Model file for the job. Use its own axes, mm. A direction names the side the tool comes from. Give positions to 0.01 mm unless a question says otherwise; leave off trailing zeros. Order: outer loops, then holes, each group sorted by start corner. A loop starts at its lowest first (then second) coordinate and runs counter-clockwise, first axis right, second up. Notation, with made-up numbers: M -40,43.25 L -2,43.25 A18 cw -2,69.25 Z; hole C -31,36.5 d4. An arc over 180 degrees is marked long. Return JSON: item names as keys, results as strings. Group by question number.
1. 3-axis set-ups, long thin cutter, end or side, ignore diameter. For faces 1 (the face through (0.33, 96.48, -19.07)), 2 (the face through (0, 41, -14)), 3 (the face through (-10, 63, -11)): which of +Z, -Z, +X, -X, +Y, -Y reach the whole face in a straight line?
2. Slice it at C-C on y = 77.5. List the corners of the cut face in (x, z).
3. Wall check: probe 1 along Y at (x, z) = (0, -3.25); probe 2 along Y at (x, z) = (0, -19.25); probe 3 along X at (y, z) = (21, -12). Give the ranges that are in metal, low to high. Write a range as [from, to].
4. Slice it at D-D on x = -4. List the corners of the cut face in (y, z).
5. Slice it at A-A on x = 0. List the corners of the cut face in (y, z).
6. Slice it at B-B on z = -17. List the corners of the cut face in (x, y), then the cut area to 3 significant figures.
7. Pin check, flat tips, straight feed: pin 1 (8 mm diameter, centred on y = 35.5, z = -10.5, fed in from +X); pin 2 (6 mm diameter, centred on x = -4.5, y = 33.5, fed in from -Z); pin 3 (3 mm diameter, centred on y = 57, z = -16.5, fed in from -X); pin 4 (4 mm diameter, centred on x = -13.5, y = 31, fed in from -Z). Stop position of each tip, or through.
8. Two-plate mould, pull along Y, no slides. Class faces 4 (the face through (0, 94, -14)), 5 (the face through (0, 0, -7)), 6 (the face through (13, 51, -6)): released by +Y, released by -Y, zero draft, split by the parting line, or undercut.
from build123d import *

# Parameters (mm, degrees)
DODANIE_WYCI_GNI_CIE1_DEPTH = 104
SZKIC2_W                    = 20
SZKIC2_H                    = 20
DODANIE_WYCI_GNI_CIE2_DEPTH = 10
SZKIC3_R                    = 2.5
WYTNIJ_WYCI_GNI_CIE1_DEPTH  = 10
SZKIC4_R                    = 1.425
WYTNIJ_WYCI_GNI_CIE2_DEPTH  = 108.782187768


with BuildPart() as part:
    # Szkic1 → Dodanie-wyciągnięcie1 (new body)
    with BuildSketch(Plane(origin=(0, 0, 0), x_dir=(1, 0, 0), z_dir=(0, 1, 0))):
        Polygon((-15, 0), (15, 0), (15, 6), (10, 6), (10, 14), (-10, 14), (-10, 6), (-15, 6), align=None)
    extrude(amount=DODANIE_WYCI_GNI_CIE1_DEPTH)

    # Szkic2 → Dodanie-wyciągnięcie2 (add)
    with BuildSketch(Plane(origin=(0, 0, -14), x_dir=(-1, 0, 0), z_dir=(0, 0, -1))):
        with Locations((0, 94)):
            Rectangle(SZKIC2_W, SZKIC2_H)
    extrude(amount=DODANIE_WYCI_GNI_CIE2_DEPTH)

    # Szkic3 → Wytnij-wyciągnięcie1 (cut)
    with BuildSketch(Plane(origin=(0, 0, -24), x_dir=(-1, 0, 0), z_dir=(0, 0, -1))):
        with Locations((0, 94)):
            Circle(SZKIC3_R)
    extrude(amount=-WYTNIJ_WYCI_GNI_CIE1_DEPTH, mode=Mode.SUBTRACT)

    # Szkic4 → Wytnij-wyciągnięcie2 (cut, through all)
    with BuildSketch(Plane.XY):
        with Locations((0, 7.425)):
            Circle(SZKIC4_R)
    extrude(amount=-WYTNIJ_WYCI_GNI_CIE2_DEPTH, mode=Mode.SUBTRACT)


solid = part.part
Result:
{
 "1": {"face 1": "-Z", "face 2": "-Z, +X, -X, -Y", "face 3": "-Z, -X, +Y, -Y"},
 "2": {"outline": "M -15,-6 L -10,-6 L -10,-14 L 10,-14 L 10,-6 L 15,-6 L 15,0 L -15,0 Z"},
 "3": {"probe 1": "y = [0, 6], [8.85, 104]", "probe 2": "y = [84, 91.5], [96.5, 104]", "probe 3": "x = [-10, 10]"},
 "4": {"outline": "M 0,-14 L 84,-14 L 84,-24 L 104,-24 L 104,0 L 0,0 Z"},
 "5": {"outline": "M 0,-14 L 6,-14 L 6,0 L 0,0 Z; M 8.85,-14 L 84,-14 L 84,-24 L 91.5,-24 L 91.5,-14 L 96.5,-14 L 96.5,-24 L 104,-24 L 104,0 L 8.85,0 Z"},
 "6": {"outline": "M -10,84 L 10,84 L 10,104 L -10,104 Z; hole C 0,94 d5", "area": "380 mm2"},
 "7": {"pin 1": "stops at x = 10", "pin 2": "stops at z = -14", "pin 3": "passes through", "pin 4": "stops at z = -6"},
 "8": {"face 4": "undercut", "face 5": "released by -Y", "face 6": "zero draft"}
}
